Print and shaded views of the part. All mm, measured from the part's lowest x, y and z. Round coordinates to 2 decimals unless told otherwise and drop trailing zeros. Order: outer loops, then holes, each group sorted by start corner. A loop starts at its lowest first (then second) coordinate and runs counter-clockwise, first axis right, second up. Notation, with made-up numbers: (54.25, -24) -> (58.25, -24) arc R18 ccw to (58.25, -8) -> close; hole circle Ø4 at (-5, -38). An arc over 180 degrees is marked (long way). Answer as CSV lines item,"result". Start each with the question number.
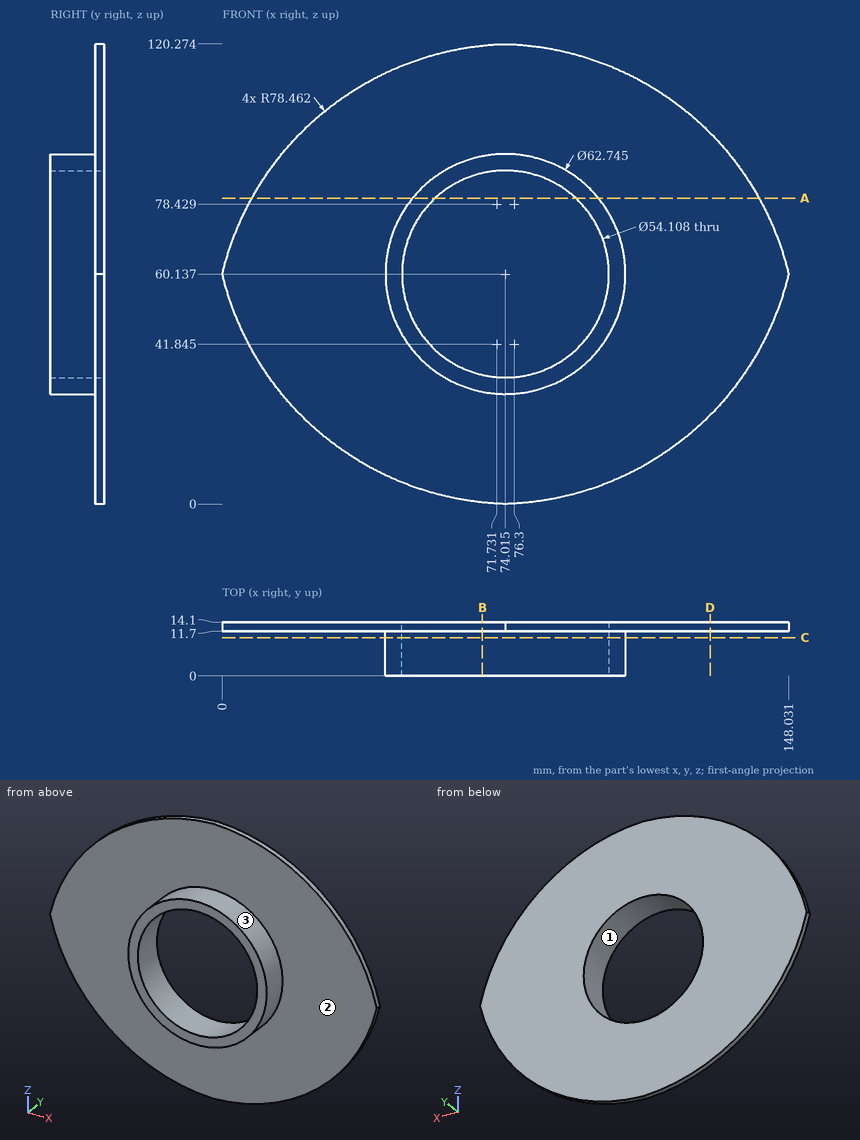
Item 1: Mould opens along Z. For the marked faces 1, 2 and 3 say: released by +Z, released by -Z, zero draft, split by the parting line, or undercut.
Item 2: Pin check, flat tips, straight feed: pin 1 (1 mm diameter, centred on x = 96, y = 6, fed in from +Z); pin 2 (8 mm diameter, centred on y = 1.5, z = 54, fed in from +X) (1 decimal); pin 3 (1.5 mm diameter, centred on x = 114.5, z = 50, fed in from -Y). Stop position of each tip, or through.
Item 3: Probe line 1 (Z direction, x = 73, y = 10.5); line 2 (Z direction, x = 74.5, y = 13.25) (1 decimal); line 3 (X direction, y = 1, z = 75.5) (1 decimal). List the from-to ranges inside material, lowest first.
Item 4: Band-saw the part on D-D, the plane x = 127.5. Give the cut face in (y, z), and give its area (3 significant figures).
Item 5: Band-saw the part on B-B, the plane x = 68. Give the cut face in (y, z).
Item 6: Band-saw the part on C-C, the plane y = 10. Give the cut face in (x, z) (1 decimal).
Item 7: Band-saw the part on A-A, the plane z = 80. Give the cut face in (x, y).
Values:
1,face 1,"undercut"
1,face 2,"zero draft"
1,face 3,"split by the parting line"
2,pin 1,"z = 83"
2,pin 2,"x = 105.3"
2,pin 3,"y = 11.7"
3,line 1,"28.78 to 33.1, 87.17 to 91.49"
3,line 2,"0 to 33.1, 87.2 to 120.3"
3,line 3,"46.7 to 51.7, 96.3 to 101.4"
4,outline,"(11.7, 23.24) -> (14.1, 23.24) -> (14.1, 97.04) -> (11.7, 97.04) -> close"
4,area,"177 mm²"
5,outline,"(0, 29.35) -> (11.7, 29.35) -> (11.7, 0.41) -> (14.1, 0.41) -> (14.1, 33.76) -> (0, 33.76) -> close; (0, 86.51) -> (14.1, 86.51) -> (14.1, 119.87) -> (11.7, 119.87) -> (11.7, 90.93) -> (0, 90.93) -> close"
6,outline,"circle Ø62.7 at (74, 60.1); hole circle Ø54.1 at (74, 60.1)"
7,outline,"(7.74, 11.7) -> (49.73, 11.7) -> (49.73, 0) -> (55.65, 0) -> (55.65, 14.1) -> (7.74, 14.1) -> close; (92.38, 0) -> (98.3, 0) -> (98.3, 11.7) -> (140.29, 11.7) -> (140.29, 14.1) -> (92.38, 14.1) -> close"
